from build123d import *

# Parameters (mm, degrees)
EXTRUDE_1_DEPTH     = 806
SKETCH_2_W          = 25
SKETCH_2_H          = 3
CUT_EXTRUDE_1_DEPTH = 26


with BuildPart() as part:
    # Эскиз1 → Вытянуть-Тонкостенный1 (new body)
    with BuildSketch(Plane(origin=(0, 0, 0), x_dir=(0, 0, -1), z_dir=(1, 0, 0))):
        Polygon((0, 25), (0, 0), (25, 0), (25, 3), (3, 3), (3, 25), align=None)
    extrude(amount=EXTRUDE_1_DEPTH)

    # Эскиз2 → Вырез-Вытянуть1 (cut, through all)
    with BuildSketch(Plane.XZ):
        with Locations((793.5, -1.5)):
            Rectangle(SKETCH_2_W, SKETCH_2_H)
        with Locations((12.5, -1.5)):
            Rectangle(SKETCH_2_W, SKETCH_2_H)
    extrude(amount=-CUT_EXTRUDE_1_DEPTH, mode=Mode.SUBTRACT)


solid = part.part
Source: CAD feature listing. Evaluate the final solid. Frame: model axes, mm. A direction names the side the tool comes from. Coordinates: 2 decimals unless noted, no trailing zeros. Loops run counter-clockwise (first coordinate to the right, second up) from the corner with the lowest first, then second, coordinate; pieces in that order, holes last. Notation, with made-up numbers: (16, 79.5) - (57, 79.5) arc R20 cw to (57, 118.5) - close; hole circle Ø2 at (-34.75, 47.25). An arc over 180 degrees is marked (long way). Return JSON: item names as keys, results as strings.
Q1. Section B-B, the plane z = -14.5. Return loops of the section in (x, y), plus the area to 3 significant figures.
Results:
{"outline": "(0, 0) - (806, 0) - (806, 3) - (0, 3) - close", "area": "2,420 mm2"}
Q2. Access query for faces 1 (the flat face through (398, 14, -3)), 2 (the flat face through (398, 13, 0)). Directions: +Z, -Z, +X, -X, +Y, -Y. A direction counts if a zero-diameter tool reaches every point of the face in a straight line with its end or side. Return the directions, or none.
Results:
{"face 1": "-Z, +X, -X, +Y", "face 2": "+Z, +X, -X, +Y, -Y"}
Q3. Contact query for flat-ended pins moving along their axis: P1, Ø3.5, axis at x = 790, y = 1, coming from the +Z side; P2, Ø12, axis at x = 195.5, z = -19, coming from the +Y side; P3, Ø1.5, axis at y = 15, z = -1, coming from the +X side. Output: stop coordinate, or through.
Results:
{"P1": "z = -3", "P2": "y = 3", "P3": "x = 781"}
Q4. Section C-C, the plane y = 8.25. Return loops of the section in (x, z), plus the area to 3 significant figures.
Results:
{"outline": "(25, -3) - (781, -3) - (781, 0) - (25, 0) - close", "area": "2,270 mm2"}
Q5. Material intervals for line 1 along Y through (x, z) = (718.5, -13); line 2 along Z through (x, y) = (386.5, 17.5); line 3 along X through (y, z) = (18.75, -2), sorted ascending.
Results:
{"line 1": "0 to 3", "line 2": "-3 to 0", "line 3": "25 to 781"}
Q6. Section A-A, the plane x = 119. Return loops of the section in (y, z), plus the area to 3 significant figures.
Results:
{"outline": "(0, -25) - (3, -25) - (3, -3) - (25, -3) - (25, 0) - (0, 0) - close", "area": "141 mm2"}
